For this review, take the finished solid that the model builds, in its own axes (mm). Face numbers are marked on the shaded views. A direction names the side the tool comes from. Coordinates: 2 decimals unless noted, no trailing zeros. Loops run counter-clockwise (first coordinate to the right, second up) from the corner with the lowest first, then second, coordinate; pieces in that order, holes last. Notation, with made-up numbers: (44, -38) -> (69, -38) arc R11 ccw to (69, -21) -> close; hole circle Ø4 at (10, 9). An arc over 180 degrees is marked (long way). Use a Markdown table: item, result.
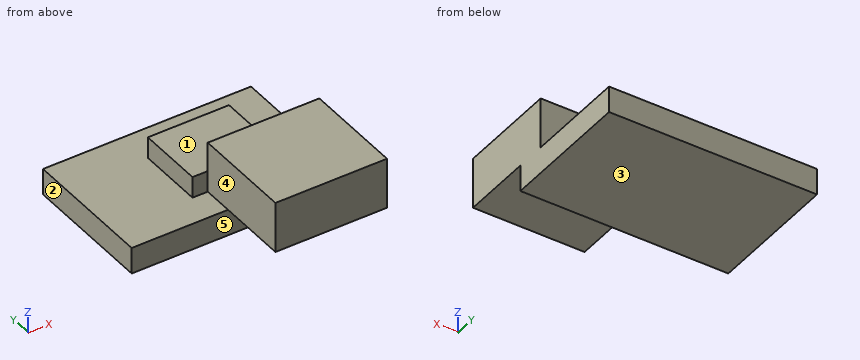
from build123d import *

# Parameters (mm, degrees)
PLACAESBOCO_W      = 20.5
PLACAESBOCO_H      = 13.1
PLACA_DEPTH        = 1.3
CONECTORESBOCO_W   = 11
CONECTORESBOCO_H   = 10
CONECTOR_DEPTH     = 5
RESISTORESESBOCO_W = 8
RESISTORESESBOCO_H = 6.6
RESISTORES_DEPTH   = 2.1


with BuildPart() as part:
    # PlacaEsboco → Placa (new, symmetric)
    with BuildSketch(Plane.XY):
        Rectangle(PLACAESBOCO_W, PLACAESBOCO_H)
    extrude(amount=PLACA_DEPTH, both=True)

    # ConectorEsboco → Conector (add)
    with BuildSketch(Plane.XY.offset(1.3)):
        with Locations((4.75, -8.55)):
            Rectangle(CONECTORESBOCO_W, CONECTORESBOCO_H)
    extrude(amount=CONECTOR_DEPTH)

    # ResistoresEsboco → Resistores (add)
    with BuildSketch(Plane.XY.offset(1.3)):
        with Locations((1.75, -0.25)):
            Rectangle(RESISTORESESBOCO_W, RESISTORESESBOCO_H)
    extrude(amount=RESISTORES_DEPTH)


solid = part.part
(1) For pin 1 Ø2 at (x, y) = (0.5, 1) entering from +Z; pin 2 Ø0.6 at (y, z) = (-1.5, 2) entering from +X; pin 3 Ø1.7 at (x, z) = (0, 3) entering from +Y, all flat-tipped, find the tip position at first contact; note any pin that passes through.
Found:
| item | result |
|---|---|
| pin 1 | stops at z = 3.4 |
| pin 2 | stops at x = 5.75 |
| pin 3 | stops at y = 3.05 |
(2) For line 1 along X through (y, z) = (-4.5, 5.75); line 2 along Z through (x, y) = (1, 4); line 3 along Y through (x, z) = (4.75, 2.75), list the stretches that pass through material, from the lowest coordinate up.
Found:
| item | result |
|---|---|
| line 1 | x = -0.75 to 10.25 |
| line 2 | z = -1.3 to 1.3 |
| line 3 | y = -13.55 to 3.05 |
(3) Take a section at D-D on z = 4.25. Write out the cut boundary in (x, y), plus the area to 3 significant figures.
Found:
| item | result |
|---|---|
| outline | (-0.75, -13.55) -> (10.25, -13.55) -> (10.25, -3.55) -> (-0.75, -3.55) -> close |
| area | 110 mm^2 |
(4) Take a section at B-B on y = -1.25. Write out the cut boundary in (x, z).
Found:
| item | result |
|---|---|
| outline | (-10.25, -1.3) -> (10.25, -1.3) -> (10.25, 1.3) -> (5.75, 1.3) -> (5.75, 3.4) -> (-2.25, 3.4) -> (-2.25, 1.3) -> (-10.25, 1.3) -> close |
(5) Take a section at C-C on x = 3.75. Write out the cut boundary in (y, z), plus the area to 3 significant figures.
Found:
| item | result |
|---|---|
| outline | (-13.55, 1.3) -> (-6.55, 1.3) -> (-6.55, -1.3) -> (6.55, -1.3) -> (6.55, 1.3) -> (3.05, 1.3) -> (3.05, 3.4) -> (-3.55, 3.4) -> (-3.55, 6.3) -> (-13.55, 6.3) -> close |
| area | 97.9 mm^2 |
(6) For the marked faces 1, 2, 3, 4 and 5, list the 3-axis set-ups (+Z, -Z, +X, -X, +Y, -Y) from which the entire face can be reached by the end or side of a thin tool; tool diameter is ignored.
Found:
| item | result |
|---|---|
| face 1 | +Z, +X, -X, +Y |
| face 2 | +Z, -Z, -X, +Y, -Y |
| face 3 | -Z, +X, -X, +Y, -Y |
| face 4 | +Z, -X, -Y |
| face 5 | -Z, +X, -X, -Y |
(7) Take a section at A-A on z = 1.75. Write out the cut boundary in (x, y), plus the area to 3 significant figures.
Found:
| item | result |
|---|---|
| outline | (-2.25, -3.55) -> (-0.75, -3.55) -> (-0.75, -13.55) -> (10.25, -13.55) -> (10.25, -3.55) -> (5.75, -3.55) -> (5.75, 3.05) -> (-2.25, 3.05) -> close |
| area | 163 mm^2 |
